```python
from build123d import *

# Parameters (mm, degrees)
F0_R     = 68.6240920578
F0_R_2   = 43.04675532
F1_DEPTH = 25.4
F3_DEPTH = 25.4
F5_COUNT = 8


with BuildPart() as f1:
    # F0 (on Front) → F1 (new body)
    with BuildSketch(Plane.XZ):
        Circle(F0_R)
        Circle(F0_R_2, mode=Mode.SUBTRACT)
    extrude(amount=F1_DEPTH)

    # F2 (on Front) → F3 (join)
    with BuildSketch(Plane.XZ):
        Polygon((10.16, 77.6048756392), (-10.16, 77.6048756392), (-17.78, 66.2807484173), (17.78, 66.2807484173), align=None)
    extrude(amount=F3_DEPTH)

    # F5: F1 ×8 about axis
    f5_axis = Axis((0, -4.3883249164, 0), (0, 1, 0))


with BuildPart() as f1_1:
    add(f1.part)
    for i in range(1, F5_COUNT):
        add(f1.part.rotate(f5_axis, i * 360 / F5_COUNT))


solid = f1_1.part
```
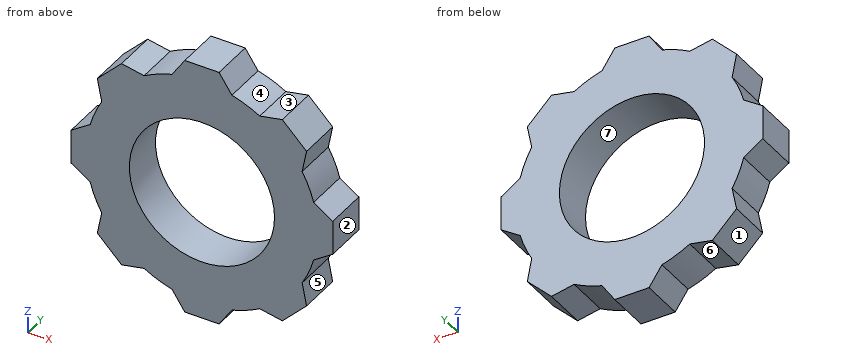
Here's how the part is built. I have some questions about the finished solid (model axes, mm). Face numbers are marked on the shaded views. A direction names the side the tool comes from. Give positions to 0.01 mm unless a question says otherwise; leave off trailing zeros. Loops run counter-clockwise (first coordinate to the right, second up) from the corner with the lowest first, then second, coordinate; pieces in that order, holes last. Notation, with made-up numbers: M 51,65.25 L 87,65.25 A30 ccw 87,100.25 Z; hole C -3.5,12.5 d7. An arc over 180 degrees is marked long. Put each result on its own line as item: value. Start each with the question number.
(1) Will these pins go through, and if not, where does the flat tip stop? pin 1 Ø4 at (x, z) = (47, -45.5) entering from +Y; pin 2 Ø1.5 at (y, z) = (-20, -29) entering from -X; pin 3 Ø3 at (y, z) = (-13, -36.5) entering from -X; pin 4 Ø4 at (x, y) = (-16, -19) entering from -Z.
(2) I need wall thicknesses on line 1 along Z through (x, y) = (0, -16); line 2 along Z through (x, y) = (39.5, -15.5). Which ranges of each line are inside material? Lowest first, please. Write a range as [from, to].
(3) I want a section at A-A on x = 0. Please give me the cut outline in (y, z), then the cut area to 3 significant figures.
(4) I want a section at D-D on x = 52.5. Please give me the cut outline in (y, z).
(5) For the marked faces 4, 5, 6 and 7, which set-ups out of +Z, -Z, +X, -X, +Y, -Y let a thin tool reach every point of the face, with its end or its side?
(6) If we mould it in two halves opening along X, with no side actions, what happens to the marked faces 1, 2 and 3? For each: +X half, -X half, draft (parallel to the pull), parting line (faces both ways), or undercut.
(7) I want a section at B-B on z = 0. Please give me the cut outline in (x, y), then the cut area to 3 significant figures.
Answer block:
1. pin 1: y = 0
1. pin 2: x = -62.54
1. pin 3: x = -60.16
1. pin 4: z = -71.9
2. line 1: [-77.6, -43.05], [43.05, 77.6]
2. line 2: [-60.46, -17.11], [17.11, 60.46]
3. outline: M -25.4,-77.6 L 0,-77.6 L 0,-43.05 L -25.4,-43.05 Z; M -25.4,43.05 L 0,43.05 L 0,77.6 L -25.4,77.6 Z
3. area: 1,760 mm^2
4. outline: M -25.4,-57.25 L 0,-57.25 L 0,57.25 L -25.4,57.25 Z
5. face 4: +Z, +Y, -Y
5. face 5: +X, +Y, -Y
5. face 6: -Z, +Y, -Y
5. face 7: +Y, -Y
6. face 1: -X half
6. face 2: +X half
6. face 3: undercut
7. outline: M -77.6,-25.4 L -43.05,-25.4 L -43.05,0 L -77.6,0 Z; M 43.05,-25.4 L 77.6,-25.4 L 77.6,0 L 43.05,0 Z
7. area: 1,760 mm^2
